```python
from build123d import *

# Parameters (mm, degrees)
F1_DEPTH = 30
F2_DEPTH = 60


with BuildPart() as f1:
    # F0 (on Front) → F1 (new body)
    with BuildSketch(Plane.XZ):
        with BuildLine():
            Line((7.7097149414, 27.9853592813), (-22.2902850586, 27.9853592813))
            Line((-22.2902850586, 27.9853592813), (-22.2902850586, 6.68e-08))
            ThreePointArc((-22.2902850586, 6.68e-08), (-7.2902850252, 15), (7.7097149414, 0))
            Line((7.7097149414, 0), (7.7097149414, 27.9853592813))
        make_face()
        with BuildLine():
            ThreePointArc((7.7097149414, 0), (-7.290285092, -15), (-22.2902850586, 6.68e-08))
            Line((-22.2902850586, 6.68e-08), (-22.2902850586, -32.0146407187))
            Line((-22.2902850586, -32.0146407187), (7.7097149414, -32.0146407187))
            Line((7.7097149414, -32.0146407187), (7.7097149414, 0))
        make_face()
        with BuildLine():
            ThreePointArc((7.7097149414, 0), (-7.2902850252, 15), (-22.2902850586, 6.68e-08))
            ThreePointArc((-22.2902850586, 6.68e-08), (-7.290285092, -15), (7.7097149414, 0))
        make_face()
    extrude(amount=F1_DEPTH)

    # F0 (on Front) → F2 (join)
    with BuildSketch(Plane.XZ):
        with BuildLine():
            ThreePointArc((7.7097149414, 0), (-7.2902850252, 15), (-22.2902850586, 6.68e-08))
            ThreePointArc((-22.2902850586, 6.68e-08), (-7.290285092, -15), (7.7097149414, 0))
        make_face()
    extrude(amount=-F2_DEPTH)


solid = f1.part
```
The listing builds one solid part. Answer for the finished solid, in the listing's coordinates (mm). A direction names the side the tool comes from. Coordinates: 2 decimals unless noted, no trailing zeros. Write each loop counter-clockwise with the first axis right and the second up, starting at its lowest first coordinate (ties: lowest second). Pieces come first, ordered by that corner, then holes.
Q1. Section A-A, the plane z = -8 is taken. Write down the section's boundary in (x, y).
Returned:
outline: (-22.29, -30) - (7.71, -30) - (7.71, 0) - (5.4, 0) - (5.4, 60) - (-19.98, 60) - (-19.98, 0) - (-22.29, 0) - close
Q2. Which of the six approach directions +Z, -Z, +X, -X, +Y, -Y give full straight-line access (tool end or side, diameter ignored) to faces 4 (the flat face through (-8, -15, -32.015)), 5 (the cylindrical face through (-21.146, 29.58, 5.745))?
Returned:
face 4: -Z, +X, -X, +Y, -Y
face 5: +Y
Q3. The mould has two halves that part along Y. Classify faces 1 (the flat face through (-8, 0, 20)), 2 (the flat face through (7.71, -15, -2)), 3 (the flat face through (-8, -30, -2)): released by +Y, released by -Y, zero draft, split by the parting line, or undercut.
Returned:
face 1: released by +Y
face 2: zero draft
face 3: released by -Y
Q4. Find the intervals of material crossed by line 1 along Y through (x, z) = (-18.75, -21); line 2 along Z through (x, y) = (-6.5, 24.5); line 3 along Z through (x, y) = (-17.25, 45), in increasing order.
Returned:
line 1: y = -30 to 0
line 2: z = -14.98 to 14.98
line 3: z = -11.22 to 11.22
Q5. Section C-C, the plane y = 22.5 is taken. Write down the section's boundary in (x, z).
Returned:
outline: circle Ø30 at (-7.29, 0)
Q6. Section D-D, the plane z = 23.5 is taken. Write down the section's boundary in (x, y), then the cut area to 3 significant figures.
Returned:
outline: (-22.29, -30) - (7.71, -30) - (7.71, 0) - (-22.29, 0) - close
area: 900 mm2
Q7. Section B-B, the plane x = -6.25 is taken. Write down the section's boundary in (y, z).
Returned:
outline: (-30, -32.01) - (0, -32.01) - (0, -14.96) - (60, -14.96) - (60, 14.96) - (0, 14.96) - (0, 27.99) - (-30, 27.99) - close
Q8. Given P1, Ø2, axis at y = 26.5, z = 12.5, coming from the +X side; P2, Ø3, axis at x = -13, y = 19.5, coming from the +Z side; P3, Ø5, axis at x = -14, y = 33.5, coming from the -Z side, each flat-ended and moving along its own axis, determine where each tip first touches the part or whether it passes through.
Returned:
P1: stops at x = 2.34
P2: stops at z = 14.4
P3: stops at z = -14.4
